```python
from build123d import *

# Parameters (mm, degrees)
BOSS_EXTRUDE1_DEPTH        = 10
CUT_EXTRUDE1_DEPTH         = 80.169628557
FILLET4_R                  = 5
CIRPATTERN6_COUNT          = 4
FILLET4_OF_CIRPATTERN6_R   = 5
FILLET5_R                  = 10
F_6_0_204_DIAMETER_HOLE1_D = 5.1816
CIRPATTERN7_COUNT          = 4


with BuildPart() as part:
    # Sketch1 → Boss-Extrude1 (new body)
    with BuildSketch(Plane(origin=(0, 0, 0), x_dir=(1, 0, 0), z_dir=(0, 1, 0))):
        Polygon((-48.461940777, 43.461940777), (-36.390872965, 55.533008589), (-29.319805153, 48.461940777), (43.461940777, 48.461940777), (55.533008589, 36.390872965), (48.461940777, 29.319805153), (48.461940777, -43.461940777), (36.390872965, -55.533008589), (29.319805153, -48.461940777), (-43.461940777, -48.461940777), (-55.533008589, -36.390872965), (-48.461940777, -29.319805153), align=None)
    extrude(amount=BOSS_EXTRUDE1_DEPTH)

    # Sketch2 → Cut-Extrude1 (cut, through all)
    with BuildSketch(Plane(origin=(0, 10, 0), x_dir=(1, 0, 0), z_dir=(0, 1, 0))):
        Polygon((-2.5, 4.571067812), (-42.426406871, -35.355339059), (-45.961940777, -31.819805153), (-45.961940777, 31.819805153), (-37.855339059, 39.926406871), align=None)
    cut_extrude1 = extrude(amount=-CUT_EXTRUDE1_DEPTH, mode=Mode.SUBTRACT)

    # Fillet4
    # the kernel refuses this fillet: 5 mm, written as the material it adds along each edge
    with BuildSketch(Plane(origin=(-37.855339059, 10, -39.926406871), x_dir=(-0.7071067811865468, 0, 0.7071067811865482), z_dir=(0, -1, 0)), Plane(origin=(-2.5, 10, -4.571067812), x_dir=(-0.7071067811865471, 0, -0.707106781186548), z_dir=(0, -1, 0))) as fillet4_piece_1:
        with BuildLine():
            CenterArc((FILLET4_R, -FILLET4_R), FILLET4_R, 90, 90)
            Line((0, -FILLET4_R), (0, 0))
            Line((0, 0), (FILLET4_R, 0))
        make_face()
    extrude(amount=10)
    with BuildSketch(Plane(origin=(-45.961940777, 10, 31.819805153), x_dir=(0.7071067811865467, 0, 0.7071067811865483), z_dir=(0, -1, 0)), Plane(origin=(-45.961940777, 10, -31.819805153), x_dir=(0, 0, 1), z_dir=(0, -1, 0))) as fillet4_piece_2:
        with BuildLine():
            CenterArc((FILLET4_R * 0.414213562373, -FILLET4_R), FILLET4_R, 90, 45)
            Line((-FILLET4_R * 0.292893218813, -FILLET4_R * 0.292893218813), (0, 0))
            Line((0, 0), (FILLET4_R * 0.414213562373, 0))
        make_face()
    extrude(amount=10)
    with BuildSketch(Plane(origin=(-42.426406871, 10, 35.355339059), x_dir=(-0.707106781186546, 0, -0.7071067811865489), z_dir=(0, -1, 0))) as fillet4_piece_3:
        with BuildLine():
            CenterArc((FILLET4_R, FILLET4_R), FILLET4_R, 180, 90)
            Line((0, FILLET4_R), (0, 0))
            Line((0, 0), (FILLET4_R, 0))
        make_face()
    extrude(amount=10)

    # CirPattern6: Cut-Extrude1 ×4 about axis
    cirpattern6_axis = Axis((0, 0, 0), (0, 1, 0))
    for i in range(1, CIRPATTERN6_COUNT):
        add(cut_extrude1.rotate(cirpattern6_axis, i * 360 / CIRPATTERN6_COUNT), mode=Mode.SUBTRACT)

    # Fillet4 of CirPattern6
    # the kernel refuses this fillet: 5 mm, written as the material it adds along each edge
    with BuildSketch(Plane(origin=(-39.926406871, 10, 37.855339059), x_dir=(0.7071067811865476, 0, -0.7071067811865476), z_dir=(0, -1, 0)), Plane(origin=(37.855339059, 10, 39.926406871), x_dir=(-0.7071067811865475, 0, -0.7071067811865475), z_dir=(0, -1, 0)), Plane(origin=(39.926406871, 10, -37.855339059), x_dir=(-0.7071067811865476, 0, 0.7071067811865476), z_dir=(0, -1, 0)), Plane(origin=(-35.355339059, 10, -42.426406871), x_dir=(0.7071067811865486, 0, -0.7071067811865465), z_dir=(0, -1, 0))) as fillet4_of_cirpattern6_piece_1:
        with BuildLine():
            CenterArc((FILLET4_OF_CIRPATTERN6_R, FILLET4_OF_CIRPATTERN6_R), FILLET4_OF_CIRPATTERN6_R, 180, 90)
            Line((0, FILLET4_OF_CIRPATTERN6_R), (0, 0))
            Line((0, 0), (FILLET4_OF_CIRPATTERN6_R, 0))
        make_face()
    extrude(amount=10)
    with BuildSketch(Plane(origin=(-4.571067812, 10, 2.5), x_dir=(-0.707106781186548, 0, 0.7071067811865469), z_dir=(0, -1, 0)), Plane(origin=(35.355339059, 10, 42.426406871), x_dir=(-0.7071067811865479, 0, -0.7071067811865471), z_dir=(0, -1, 0)), Plane(origin=(2.5, 10, 4.571067812), x_dir=(0.7071067811865474, 0, 0.7071067811865478), z_dir=(0, -1, 0)), Plane(origin=(42.426406871, 10, -35.355339059), x_dir=(-0.7071067811865471, 0, 0.7071067811865479), z_dir=(0, -1, 0)), Plane(origin=(4.571067812, 10, -2.5), x_dir=(0.7071067811865478, 0, -0.7071067811865472), z_dir=(0, -1, 0))) as fillet4_of_cirpattern6_piece_2:
        with BuildLine():
            CenterArc((FILLET4_OF_CIRPATTERN6_R, -FILLET4_OF_CIRPATTERN6_R), FILLET4_OF_CIRPATTERN6_R, 90, 90)
            Line((0, -FILLET4_OF_CIRPATTERN6_R), (0, 0))
            Line((0, 0), (FILLET4_OF_CIRPATTERN6_R, 0))
        make_face()
    extrude(amount=10)
    with BuildSketch(Plane(origin=(31.819805153, 10, 45.961940777), x_dir=(-1, 0, 0), z_dir=(0, -1, 0)), Plane(origin=(-31.819805153, 10, 45.961940777), x_dir=(-0.7071067811865483, 0, -0.7071067811865467), z_dir=(0, -1, 0)), Plane(origin=(45.961940777, 10, -31.819805153), x_dir=(0, 0, 1), z_dir=(0, -1, 0)), Plane(origin=(45.961940777, 10, 31.819805153), x_dir=(-0.7071067811865458, 0, 0.7071067811865492), z_dir=(0, -1, 0)), Plane(origin=(-31.819805153, 10, -45.961940777), x_dir=(1, 0, 0), z_dir=(0, -1, 0)), Plane(origin=(31.819805153, 10, -45.961940777), x_dir=(0.7071067811865492, 0, 0.7071067811865458), z_dir=(0, -1, 0))) as fillet4_of_cirpattern6_piece_3:
        with BuildLine():
            CenterArc((FILLET4_OF_CIRPATTERN6_R * 0.414213562373, FILLET4_OF_CIRPATTERN6_R), FILLET4_OF_CIRPATTERN6_R, 225, 45)
            Line((-FILLET4_OF_CIRPATTERN6_R * 0.292893218813, FILLET4_OF_CIRPATTERN6_R * 0.292893218813), (0, 0))
            Line((0, 0), (FILLET4_OF_CIRPATTERN6_R * 0.414213562373, 0))
        make_face()
    extrude(amount=10)

    # Fillet5
    fillet5_edges = [part.edges().sort_by_distance(p)[0] for p in [
        (-48.461940777, 5, -43.461940777),
        (-29.319805153, 5, -48.461940777),
        (43.461940777, 5, -48.461940777),
        (48.461940777, 5, -29.319805153),
        (48.461940777, 5, 43.461940777),
        (29.319805153, 5, 48.461940777),
        (-43.461940777, 5, 48.461940777),
        (-48.461940777, 5, 29.319805153),
    ]]
    fillet(fillet5_edges, radius=FILLET5_R)

    # #6 (0.204) Diameter Hole1 (through all)
    with Locations(Plane(origin=(0, 10, 0), x_dir=(1, 0, 0), z_dir=(0, 1, 0))):
        with Locations((-42.426406871, 42.426406871), (-36.390872965, 48.461940777)):
            f_6_0_204_diameter_hole1 = Hole(F_6_0_204_DIAMETER_HOLE1_D / 2)

    # CirPattern7: #6 (0.204) Diameter Hole1 ×4 about axis
    cirpattern7_axis = Axis((0, 0, 0), (0, 1, 0))
    for i in range(1, CIRPATTERN7_COUNT):
        add(f_6_0_204_diameter_hole1.rotate(cirpattern7_axis, i * 360 / CIRPATTERN7_COUNT), mode=Mode.SUBTRACT)


solid = part.part
```
Geometry: final body of the model. Coordinates: model frame, mm. A direction names the side the tool comes from. Coordinates: 2 decimals unless noted, no trailing zeros. Order: outer loops, then holes, each group sorted by start corner. A loop starts at its lowest first (then second) coordinate and runs counter-clockwise, first axis right, second up. Notation, with made-up numbers: (55, -9) -> (85, -9) arc R13 cw to (85, -4) -> close; hole circle Ø7 at (-33.5, 0). An arc over 180 degrees is marked (long way). Write item = value, one per line.
(1) Cut plane C-C on y = 7.75. Count the separate pieces of the cut face and the enclosed holes in it, plus the area to 3 significant figures.
Solved:
separate_pieces = 1
enclosed_holes = 12
area = 2,200 mm²
(2) Cut plane A-A on z = 14.5. Return loops of the section in (x, y).
Solved:
outline = (-48.46, 0) -> (-45.96, 0) -> (-45.96, 10) -> (-48.46, 10) -> close; (-21.57, 0) -> (-16.57, 0) -> (-16.57, 10) -> (-21.57, 10) -> close; (7.43, 0) -> (12.43, 0) -> (12.43, 10) -> (7.43, 10) -> close; (45.96, 0) -> (48.46, 0) -> (48.46, 10) -> (45.96, 10) -> close
(3) Pin query (flat end, axial travel): pin 1 Ø5 at (y, z) = (7, -0.5) entering from +X; pin 2 Ø3 at (x, y) = (-10.5, 6.5) entering from +Z; pin 3 Ø3 at (y, z) = (5, 12.5) entering from -X; pin 4 Ø4 at (x, z) = (36.39, 48.46) entering from -Y. Return the tip coordinate at first contact, or that it passes through.
Solved:
pin_1 = 48.46
pin_2 = 48.46
pin_3 = -48.46
pin_4 = through
(4) Pull-direction query (Z, two-part tool) for faces 1 (the flat face through (7, 5, -48.462)), 2 (the flat face through (45.962, 5, 0)), 3 (the flat face through (34.35, 4.93, 53.49)); classes: pulls with the +Z half, pulls with the -Z half, needs draft (parallel to the pull), parting line crosses it, or undercut.
Solved:
face_1 = pulls with the -Z half
face_2 = undercut
face_3 = pulls with the +Z half
(5) Access query for faces 4 (the flat face through (-4, 10, -3)), 5 (the cylindrical face through (-4.63, 5.07, 4.57)). Directions: +Z, -Z, +X, -X, +Y, -Y. A direction counts if a zero-diameter tool reaches every point of the face in a straight line with its end or side. Return the directions, or none.
Solved:
face_4 = +Z, -Z, +X, -X, +Y
face_5 = +Y, -Y
(6) Line query: line 1 (X direction, y = 4.25, z = 13); line 2 (X direction, y = 6, z = -34.5); line 3 (Z direction, x = 22, y = 9.75). Output: solid intervals per line, ascending.
Solved:
line_1 = -48.46 to -45.96, -20.07 to -15.07, 5.93 to 10.93, 45.96 to 48.46
line_2 = -48.46 to -43.28, -32.43 to -27.43, 36.56 to 46.69, 50.23 to 53.64
line_3 = -48.46 to -45.96, -19.93 to -14.93, 24.07 to 29.07, 45.96 to 48.46
(7) Cut plane B-B on x = 22. Return loops of the section in (y, z).
Solved:
outline = (0, -48.46) -> (10, -48.46) -> (10, -45.96) -> (0, -45.96) -> close; (0, -19.93) -> (10, -19.93) -> (10, -14.93) -> (0, -14.93) -> close; (0, 24.07) -> (10, 24.07) -> (10, 29.07) -> (0, 29.07) -> close; (0, 45.96) -> (10, 45.96) -> (10, 48.46) -> (0, 48.46) -> close
